The listing builds one solid part. Answer for the finished solid, in the listing's coordinates (mm). Face numbers are marked on the shaded views. A direction names the side the tool comes from. Give positions to 0.01 mm unless a question says otherwise; leave off trailing zeros. Loops run counter-clockwise (first coordinate to the right, second up) from the corner with the lowest first, then second, coordinate; pieces in that order, holes last.
Item 1: Section D-D, the plane z = -8 is taken. Give the vertices of the cut face in (x, y).
Item 2: Each of these flat-tipped pins is pushed along its axis until it touches: pin 1 Ø24 at (x, y) = (-18, -34) entering from +Z; pin 2 Ø6 at (y, z) = (6, 27.5) entering from -X; pin 3 Ø1 at (x, z) = (-30, 33) entering from -Y (3 decimals); pin 4 Ø6 at (y, z) = (23, 28.5) entering from -X. Where does it stop, or does it pass through?
Item 3: Consider line 1 along Z through (x, y) = (-28, -37.5); line 2 along X through (y, z) = (3, 0); line 3 along Y through (x, z) = (-0.5, 29) (3 decimals). Determine where each line is inside the solid, lowest interval first.
Item 4: Section B-B, the plane z = 19 is taken. Give the vertices of the cut face in (x, y) (3 decimals).
Item 5: Section C-C, the plane x = 96 is taken. Give the vertices of the cut face in (y, z) (3 decimals), and give its area (3 significant figures).
Item 6: Section A-A, the plane y = -32.5 is taken. Give the vertices of the cut face in (x, z), and give its area (3 significant figures).
Item 7: A tool of negligible diameter and unlimited length cuts with its end or side. For the marked faces 1, 2, 3, 4 and 5, from which of +Z, -Z, +X, -X, +Y, -Y can it reach the whole face along a straight path? Write none if from no direction.
from build123d import *

# Parameters (mm, degrees)
F1_DEPTH = 63.5
F2_DEPTH = 12.7
F3_DEPTH = 3.175
F4_R     = 12.7


with BuildPart() as f1:
    # F0 (on Front) → F1 (new body, symmetric)
    with BuildSketch(Plane.XZ):
        Polygon((32.4870109211, 25.4), (-50.8, 25.4), (-50.8, -25.4), (50.8, -25.4), (50.8, 25.4), align=None)
    extrude(amount=F1_DEPTH, both=True)

    # F0 (on Front) → F2 (join, symmetric)
    with BuildSketch(Plane.XZ):
        with BuildLine():
            Line((32.4870109211, 33.1416912377), (32.4870109211, 25.4))
            Line((32.4870109211, 25.4), (50.8, 25.4))
            Line((50.8, 25.4), (50.8, 33.1416912377))
            ThreePointArc((50.8, 33.1416912377), (54.5197438789, 42.1219473588), (63.5, 45.8416912377))
            Line((63.5, 45.8416912377), (67.4773146418, 45.8416912377))
            Line((67.4773146418, 45.8416912377), (67.4773146418, 64.1546803166))
            Line((67.4773146418, 64.1546803166), (63.5, 64.1546803166))
            add(Edge.make_bspline(
                [(60.7238640338, 64.0301771298), (61.6427833631, 64.0736819476), (62.5681528274, 64.1151925709), (63.5, 64.1546803166)],
                knots=[119.3459466449, 119.3459466449, 119.3459466449, 119.3459466449, 120.6914050231, 120.6914050231, 120.6914050231, 120.6914050231], degree=3))
            ThreePointArc((60.7238640338, 64.0301771298), (40.6100265836, 54.066666951), (32.4870109211, 33.1416912377))
        make_face()
    extrude(amount=F2_DEPTH, both=True)

    # F0 (on Front) → F3 (join, symmetric)
    with BuildSketch(Plane.XZ):
        with BuildLine():
            add(Edge.make_bspline(
                [(-50.8, 25.4), (-51.5467154079, 40.6214778369), (-20.7868679356, 60.1711772937), (60.7238640338, 64.0301771298)],
                knots=[0, 0, 0, 0, 119.3459466449, 119.3459466449, 119.3459466449, 119.3459466449], degree=3))
            Line((-50.8, 25.4), (32.4870109211, 25.4))
            Line((32.4870109211, 25.4), (32.4870109211, 33.1416912377))
            ThreePointArc((32.4870109211, 33.1416912377), (40.6100265836, 54.066666951), (60.7238640338, 64.0301771298))
        make_face()
        Polygon((32.4870109211, 25.4), (-50.8, 25.4), (-50.8, -25.4), (50.8, -25.4), (50.8, 25.4), align=None)
        with BuildLine():
            Line((32.4870109211, 33.1416912377), (32.4870109211, 25.4))
            Line((32.4870109211, 25.4), (50.8, 25.4))
            Line((50.8, 25.4), (50.8, 33.1416912377))
            ThreePointArc((50.8, 33.1416912377), (54.5197438789, 42.1219473588), (63.5, 45.8416912377))
            Line((63.5, 45.8416912377), (67.4773146418, 45.8416912377))
            Line((67.4773146418, 45.8416912377), (67.4773146418, 64.1546803166))
            Line((67.4773146418, 64.1546803166), (63.5, 64.1546803166))
            add(Edge.make_bspline(
                [(60.7238640338, 64.0301771298), (61.6427833631, 64.0736819476), (62.5681528274, 64.1151925709), (63.5, 64.1546803166)],
                knots=[119.3459466449, 119.3459466449, 119.3459466449, 119.3459466449, 120.6914050231, 120.6914050231, 120.6914050231, 120.6914050231], degree=3))
            ThreePointArc((60.7238640338, 64.0301771298), (40.6100265836, 54.066666951), (32.4870109211, 33.1416912377))
        make_face()
        with BuildLine():
            ThreePointArc((63.5, 64.1546803166), (62.1105367991, 64.1235388847), (60.7238640338, 64.0301771298))
            add(Edge.make_bspline(
                [(60.7238640338, 64.0301771298), (61.6427833631, 64.0736819476), (62.5681528274, 64.1151925709), (63.5, 64.1546803166)],
                knots=[119.3459466449, 119.3459466449, 119.3459466449, 119.3459466449, 120.6914050231, 120.6914050231, 120.6914050231, 120.6914050231], degree=3))
        make_face()
        Polygon((67.4773146418, 64.4600404125), (67.4773146418, 64.1546803166), (67.4773146418, 45.8416912377), (67.4773146418, 39.0600404125), (118.2773146418, 39.0600404125), (118.2773146418, 64.4600404125), align=None)
    extrude(amount=F3_DEPTH, both=True)

    # F4
    f4_edges = [f1.edges().sort_by_distance(p)[0] for p in [
        (-50.8, 33.3375, 25.4),
        (0, 63.5, 25.4),
        (50.8, 38.1, 25.4),
        (0, -63.5, 25.4),
        (50.8, -38.1, 25.4),
        (-50.8, -33.3375, 25.4),
        (-50.8, 63.5, 0),
    ]]
    fillet(f4_edges, radius=F4_R)


solid = f1.part
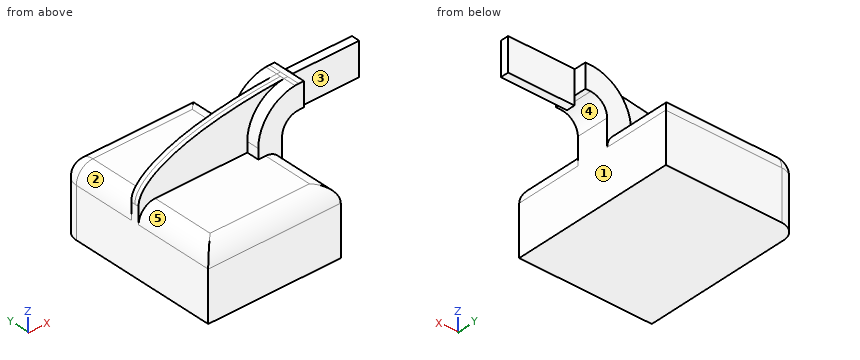
Worked answers:
1. outline: (-50.8, -63.5) - (50.8, -63.5) - (50.8, 63.5) - (-38.1, 63.5) arc R12.7 ccw to (-50.8, 50.8) - close
2. pin 1: stops at z = 25.4
2. pin 2: stops at x = -50.8
2. pin 3: stops at y = -3.175
2. pin 4: passes through
3. line 1: z = -25.4 to 25.4
3. line 2: x = -50.8 to 50.8
3. line 3: y = -3.175 to 3.175
4. outline: (-50.8, -3.175) - (-49.127, -3.175) - (-49.127, -61.827) - (49.127, -61.827) - (49.127, -12.7) - (50.8, -12.7) - (50.8, 12.7) - (49.127, 12.7) - (49.127, 61.827) - (-38.1, 61.827) arc R11.027 ccw to (-49.127, 50.8) - (-49.127, 3.175) - (-50.8, 3.175) - close
5. outline: (-3.175, 39.06) - (3.175, 39.06) - (3.175, 64.46) - (-3.175, 64.46) - close
5. area: 161 mm2
6. outline: (-50.8, -25.4) - (50.8, -25.4) - (50.8, 12.7) arc R12.7 ccw to (38.1, 25.4) - (-38.1, 25.4) arc R12.7 ccw to (-50.8, 12.7) - close
6. area: 5,090 mm2
7. face 1: -Z, +X, +Y, -Y
7. face 2: +Z, -X, +Y
7. face 3: +Z, -Z, +X, -Y
7. face 4: -Z, +Y, -Y
7. face 5: +Z, -X, -Y
